Here's how the part is built. I have some questions about the finished solid (model axes, mm). Face numbers are marked on the shaded views. A direction names the side the tool comes from. Round coordinates to 2 decimals unless told otherwise and drop trailing zeros. Loops run counter-clockwise (first coordinate to the right, second up) from the corner with the lowest first, then second, coordinate; pieces in that order, holes last. Notation, with made-up numbers: M 10.25,22 L 34.25,22 A14 ccw 34.25,48 Z; hole C 42.25,52 d5. An arc over 180 degrees is marked long. Answer as a JSON object with one key per item and string values.
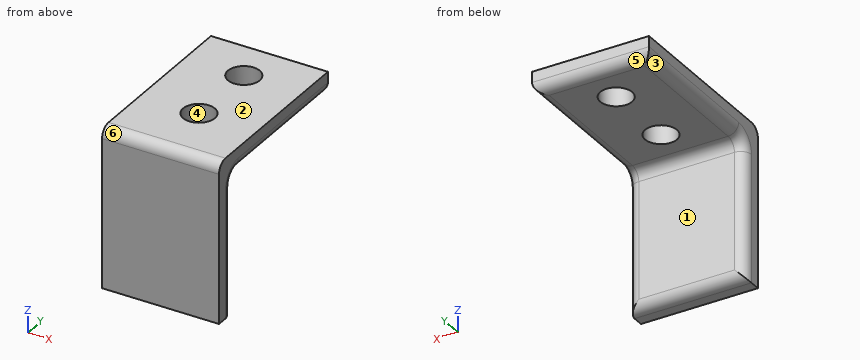
from build123d import *

# Parameters (mm, degrees)
ESBO_O1_W                = 11
ESBO_O1_H                = 19
RESSALTO_EXTRUS_O1_DEPTH = 2
ESBO_O2_W                = 11
ESBO_O2_H                = 2
RESSALTO_EXTRUS_O2_DEPTH = 15
ESBO_O3_R                = 1.5
CORTE_EXTRUS_O1_DEPTH    = 15
ESBO_O4_W                = 11
ESBO_O4_H                = 4
CORTE_EXTRUS_O2_DEPTH    = 15
FILETE1_R                = 1
FILETE2_R                = 1


with BuildPart() as part:
    # Esboço1 → Ressalto-extrusão1 (new body)
    with BuildSketch(Plane(origin=(0, 0, 0), x_dir=(1, 0, 0), z_dir=(0, 1, 0))):
        with Locations((-25.942415051, -17.124578687)):
            Rectangle(ESBO_O1_W, ESBO_O1_H)
    extrude(amount=RESSALTO_EXTRUS_O1_DEPTH)

    # Esboço2 → Ressalto-extrusão2 (add)
    with BuildSketch(Plane(origin=(0, 2, 0), x_dir=(1, 0, 0), z_dir=(0, 1, 0))):
        with Locations((-25.942415051, -25.624578687)):
            Rectangle(ESBO_O2_W, ESBO_O2_H)
    extrude(amount=RESSALTO_EXTRUS_O2_DEPTH)

    # Esboço3 → Corte-extrusão1 (cut)
    with BuildSketch(Plane(origin=(0, 0, 24.624578687), x_dir=(-1, 0, 0), z_dir=(0, 0, -1))):
        with Locations((25.942415051, 6)):
            Circle(ESBO_O3_R)
        with Locations((25.942415051, 13)):
            Circle(ESBO_O3_R)
    extrude(amount=-CORTE_EXTRUS_O1_DEPTH, mode=Mode.SUBTRACT)

    # Esboço4 → Corte-extrusão2 (cut)
    with BuildSketch(Plane(origin=(0, 2, 0), x_dir=(1, 0, 0), z_dir=(0, 1, 0))):
        with Locations((-25.942415051, -9.624578687)):
            Rectangle(ESBO_O4_W, ESBO_O4_H)
    extrude(amount=-CORTE_EXTRUS_O2_DEPTH, mode=Mode.SUBTRACT)

    # Filete1
    filete1_edges = [part.edges().sort_by_distance(p)[0] for p in [
        (-25.942415051, 2, 24.624578687),
        (-25.942415051, 0, 26.624578687),
    ]]
    fillet(filete1_edges, radius=FILETE1_R)

    # Filete2
    filete2_edges = [part.edges().sort_by_distance(p)[0] for p in [
        (-31.442415051, 10, 24.624578687),
        (-20.442415051, 10, 24.624578687),
        (-25.942415051, 17, 24.624578687),
        (-31.442415051, 2, 17.624578687),
        (-25.942415051, 2, 11.624578687),
        (-20.442415051, 2, 17.624578687),
        (-31.442415051, 2.292893219, 24.331685469),
        (-20.442415051, 2.292893219, 24.331685469),
    ]]
    fillet(filete2_edges, radius=FILETE2_R)


solid = part.part
Item 1: If I drill on L1, parallel to Y at x = -27.5, z = 16.5; L2, parallel to Z at x = -24.25, y = 13; L3, parallel to Y at x = -25, z = 26.25, over which ranges is the centre line in solid material (lowest first)? Write a range as from..to.
Solution:
{"L1": "y = 0..2", "L2": "z = 24.62..26.62", "L3": "y = 0.22..4.83, 7.17..11.83, 14.17..17"}
Item 2: I want a section at C-C on x = -25.75. List the corners of the cut face in (y, z) for me, plus the area to 3 significant figures.
Solution:
{"outline": "M 0,11.62 L 1,11.62 A1 ccw 2,12.62 L 2,23.62 A1 cw 3,24.62 L 4.51,24.62 L 4.51,26.62 L 1,26.62 A1 ccw 0,25.62 Z; M 7.49,24.62 L 11.51,24.62 L 11.51,26.62 L 7.49,26.62 Z; M 14.49,24.62 L 16,24.62 A1 ccw 17,25.62 L 17,26.62 L 14.49,26.62 Z", "area": "47.7 mm2"}
Item 3: We'd pull the mould along Y, two halves only. Please class the marked faces 4, 5 and 6: +Y half, -Y half, draft (parallel to the pull), parting line (faces both ways), or undercut.
Solution:
{"face 4": "undercut", "face 5": "+Y half", "face 6": "-Y half"}
Item 4: I want a section at A-A on y = 6. List the corners of the cut face in (x, z) for me, plus the area to 3 significant figures.
Solution:
{"outline": "M -31.44,25.62 A1 ccw -30.44,24.62 L -27.44,24.62 L -27.44,26.62 L -31.44,26.62 Z; M -24.44,24.62 L -21.44,24.62 A1 ccw -20.44,25.62 L -20.44,26.62 L -24.44,26.62 Z", "area": "15.6 mm2"}
Item 5: For P1, Ø1, axis at x = -27, y = 14.5, coming from the -Z side; P2, Ø2, axis at x = -25.5, z = 13.5, coming from the +Y side; P3, Ø1.5, axis at x = -25, z = 24.5, coming from the +Y side, each with a flat end and sliding along its axis, tell me the tip position at first contact or that it passes through.
Solution:
{"P1": "stops at z = 24.62", "P2": "stops at y = 2", "P3": "stops at y = 16.93"}
Item 6: I want a section at B-B on z = 22. List the corners of the cut face in (x, y) for me.
Solution:
{"outline": "M -31.44,0 L -20.44,0 L -20.44,1 A1 ccw -21.44,2 L -30.44,2 A1 ccw -31.44,1 Z"}
Item 7: I want a section at D-D on x = -29.5. List the corners of the cut face in (y, z) for me, plus the area to 3 significant figures.
Solution:
{"outline": "M 0,11.62 L 1,11.62 A1 ccw 2,12.62 L 2,23.62 A1 cw 3,24.62 L 16,24.62 A1 ccw 17,25.62 L 17,26.62 L 1,26.62 A1 ccw 0,25.62 Z", "area": "59.6 mm2"}
Item 8: For the marked faces 1, 2 and 3, which set-ups out of +Z, -Z, +X, -X, +Y, -Y let a thin tool reach every point of the face, with its end or its side?
Solution:
{"face 1": "-Z, +X, -X, +Y", "face 2": "+Z, +X, -X, +Y, -Y", "face 3": "-Z, -X, +Y"}
